Here's how the part is built. I have some questions about the finished solid (model axes, mm). A direction names the side the tool comes from. Give positions to 0.01 mm unless a question says otherwise; leave off trailing zeros. Order: outer loops, then holes, each group sorted by start corner. A loop starts at its lowest first (then second) coordinate and runs counter-clockwise, first axis right, second up. Notation, with made-up numbers: (7.5, 25.5) -> (63.5, 25.5) arc R14 cw to (63.5, 32.5) -> close; hole circle Ø1 at (89.5, -26). An arc over 180 degrees is marked (long way). Write each question's results on one line, items separated by ' | '. Start each with the question number.
Q1. Imagine slicing it at C-C, the plane z = -10.75. Please give me the cut outline in (x, y).
Q2. For faces 4 (the face through (-100, 111, -12.7)), 5 (the face through (-98, 98, -3.175)), which set-ups out of +Z, -Z, +X, -X, +Y, -Y let a thin tool reach every point of the face, with its end or its side?
Q3. I need wall thicknesses on line 1 along Y through (x, z) = (0, -0.7); line 2 along X through (y, z) = (-75.5, -8.25); line 3 along X through (y, z) = (30, -12). Which ranges of each line are inside material? Lowest first, please. Write a range as [from, to].
Q4. Thinking about a two-plate mould opening in Y: for faces 1 (the face through (122, 66, 0)), 2 (the face through (-109.55, 84, -1.61)), 3 (the face through (81.042, -127.112, -6.261)), which applies, pulls with the +Y half, pulls with the -Y half, needs draft (parallel to the pull), parting line crosses it, or undercut?
Q5. Imagine slicing it at B-B, the plane x = -68.5. Please give me the cut outline in (y, z) (3 decimals).
Q6. I'm going to push flat-ended pins straight in: pin 1 (2 mm diameter, centred on y = -74, z = -2, fed in from +X); pin 2 (2 mm diameter, centred on y = -114, z = -2, fed in from -X); pin 3 (3 mm diameter, centred on x = -83.47, y = -114.88, fed in from -Z) (3 decimals). Where does each tip first touch, or does it pass through?
Q7. Imagine slicing it at A-A, the plane y = -79. Please give me the cut outline in (x, z) (3 decimals).
```python
from build123d import *

# Parameters (mm, degrees)
F_4_40_TAPPED_HOLE1_D = 2.2606
CIRPATTERN1_COUNT     = 10


with BuildPart() as part:
    # Sketch1 → Revolve1 (revolve)
    with BuildSketch(Plane(origin=(0, 0, 0), x_dir=(0, 0, -1), z_dir=(1, 0, 0)), mode=Mode.PRIVATE) as revolve1_sk:
        Polygon((3.175, 147.574), (12.7, 147.574), (12.7, 150.749), (0, 150.749), (0, 138.049), (3.175, 138.049), align=None)
    revolve(revolve1_sk.sketch.rotate(Axis((0, 0, 0), (0, 0, -1)), 90), axis=Axis((0, 0, 0), (0, 0, -1)))

    # #4-40 Tapped Hole1 (through all)
    with Locations(Plane.XY):
        with Locations((0, 142)):
            f_4_40_tapped_hole1 = Hole(F_4_40_TAPPED_HOLE1_D / 2)

    # CirPattern1: #4-40 Tapped Hole1 ×10 about axis
    cirpattern1_axis = Axis((0, 0, 0), (0, 0, 1))
    for i in range(1, CIRPATTERN1_COUNT):
        add(f_4_40_tapped_hole1.rotate(cirpattern1_axis, i * 360 / CIRPATTERN1_COUNT), mode=Mode.SUBTRACT)


solid = part.part
```
Geometry check:
1) outline: circle Ø301.5 at (0, 0); hole circle Ø295.15 at (0, 0)
2) face 4: -Z, +X, -X, +Y, -Y | face 5: -Z
3) line 1: [-150.75, -143.13], [-140.87, -138.05], [138.05, 140.87], [143.13, 150.75] | line 2: [-130.48, -126.8], [126.8, 130.48] | line 3: [-147.73, -144.49], [144.49, 147.73]
4) face 1: needs draft | face 2: undercut | face 3: parting line crosses it
5) outline: (-134.287, -12.7) -> (-130.713, -12.7) -> (-130.713, -3.175) -> (-119.855, -3.175) -> (-119.855, 0) -> (-134.287, 0) -> close; (119.855, -3.175) -> (130.713, -3.175) -> (130.713, -12.7) -> (134.287, -12.7) -> (134.287, 0) -> (119.855, 0) -> close
6) pin 1: x = 131.89 | pin 2: x = -99.78 | pin 3: z = -3.175
7) outline: (-128.391, -12.7) -> (-124.648, -12.7) -> (-124.648, -3.175) -> (-113.21, -3.175) -> (-113.21, 0) -> (-128.391, 0) -> close; (113.21, -3.175) -> (124.648, -3.175) -> (124.648, -12.7) -> (128.391, -12.7) -> (128.391, 0) -> (113.21, 0) -> close
